```python
from build123d import *

# Parameters (mm, degrees)
SKETCH2_R                        = 3
BOSS_EXTRUDE1_DEPTH              = 25
SKETCH5_W                        = 200
SKETCH5_H                        = 44
CUT_EXTRUDE1_DEPTH               = 8
SENSORMODULE_BOTTOMMIDDLEE_DEPTH = 4.5
SKETCH12_W                       = 247.875067181
SKETCH12_H                       = 102.432022038
CUT_EXTRUDE2_DEPTH               = 14
SKETCH14_W                       = 9.40210165
SKETCH14_H                       = 8
SKETCH14_W_2                     = 8.199489831
BOSS_EXTRUDE2_DEPTH              = 48
FILLET1_R                        = 3
FILLET2_R                        = 3
SKETCH15_W                       = 3.793616894
SKETCH15_H                       = 8.666666667
SKETCH15_H_2                     = 8.666666666
BOSS_EXTRUDE3_DEPTH              = 8
SKETCH16_W                       = 3.793616895
SKETCH16_H                       = 8.666666667
SKETCH16_H_2                     = 8.666666666
BOSS_EXTRUDE4_DEPTH              = 10


with BuildPart() as part:
    # Sketch2 → Boss-Extrude1 (new body)
    with BuildSketch(Plane(origin=(0, 0, 0), x_dir=(1, 0, 0), z_dir=(0, 1, 0))):
        with BuildLine():
            Line((-33, -35), (33, -35))
            ThreePointArc((33, -35), (36.535533906, -33.535533906), (38, -30))
            Line((38, -30), (38, 30))
            ThreePointArc((38, 30), (36.535533906, 33.535533906), (33, 35))
            Line((33, 35), (-33, 35))
            ThreePointArc((-33, 35), (-36.535533906, 33.535533906), (-38, 30))
            Line((-38, 30), (-38, -30))
            ThreePointArc((-38, -30), (-36.535533906, -33.535533906), (-33, -35))
        make_face()
        with Locations((-33, 30)):
            Circle(SKETCH2_R, mode=Mode.SUBTRACT)
        with Locations((-33, -30)):
            Circle(SKETCH2_R, mode=Mode.SUBTRACT)
        with Locations((33, 30)):
            Circle(SKETCH2_R, mode=Mode.SUBTRACT)
        with Locations((33, -30)):
            Circle(SKETCH2_R, mode=Mode.SUBTRACT)
    extrude(amount=BOSS_EXTRUDE1_DEPTH)

    # Sketch5 → Cut-Extrude1 (cut)
    with BuildSketch(Plane(origin=(0, 25, 0), x_dir=(1, 0, 0), z_dir=(0, 1, 0))):
        Rectangle(SKETCH5_W, SKETCH5_H)
    extrude(amount=-CUT_EXTRUDE1_DEPTH, mode=Mode.SUBTRACT)

    # Sketch6 → SensorModule(bottomMiddlee) (add)
    with BuildSketch(Plane(origin=(87.622938947, 17, 0), x_dir=(1, 0, 0), z_dir=(0, 1, 0))):
        Polygon((-106.839454309, 15.5), (-75.839454309, 15.5), (-75.839454309, 7.8), (-68.839454309, 7.8), (-68.839454309, -7.4), (-75.839454309, -7.4), (-75.839454309, -15.5), (-106.839454309, -15.5), align=None)
    extrude(amount=SENSORMODULE_BOTTOMMIDDLEE_DEPTH)

    # Sketch12 → Cut-Extrude2 (cut)
    with BuildSketch(Plane.XZ):
        with Locations((-0.926975658, -6.36803857)):
            Rectangle(SKETCH12_W, SKETCH12_H)
    extrude(amount=-CUT_EXTRUDE2_DEPTH, mode=Mode.SUBTRACT)

    # Sketch14 → Boss-Extrude2 (add)
    with BuildSketch(Plane.XY.offset(-22)):
        with Locations((-33.298949175, 21)):
            Rectangle(SKETCH14_W, SKETCH14_H)
        with Locations((33.900255085, 21)):
            Rectangle(SKETCH14_W_2, SKETCH14_H)
    extrude(amount=BOSS_EXTRUDE2_DEPTH)

    # Fillet1
    fillet1_edges = [part.edges().sort_by_distance(p)[0] for p in [
        (0.601305909, 17, -22),
    ]]
    fillet(fillet1_edges, radius=FILLET1_R)

    # Fillet2
    fillet2_edges = [part.edges().sort_by_distance(p)[0] for p in [
        (0.601305909, 17, 22),
    ]]
    fillet(fillet2_edges, radius=FILLET2_R)

    # Sketch15 → Boss-Extrude3 (add)
    with BuildSketch(Plane(origin=(3.489394794, 17, 0), x_dir=(1, 0, 0), z_dir=(0, 1, 0))):
        with Locations((-27.729371665, 12.666666666)):
            Rectangle(SKETCH15_W, SKETCH15_H)
        with Locations((-27.729371665, 0)):
            Rectangle(SKETCH15_W, SKETCH15_H_2)
        with Locations((-27.729371665, -12.666666666)):
            Rectangle(SKETCH15_W, SKETCH15_H)
    extrude(amount=BOSS_EXTRUDE3_DEPTH)

    # Sketch16 → Boss-Extrude4 (add)
    with BuildSketch(Plane(origin=(51.94610351, 25, 9.710186869), x_dir=(1, 0, 0), z_dir=(0, 1, 0))):
        with Locations((-27.906397887, 22.722574296)):
            Rectangle(SKETCH16_W, SKETCH16_H)
        with Locations((-27.906397887, 10.055907629)):
            Rectangle(SKETCH16_W, SKETCH16_H_2)
        with Locations((-27.906397887, -2.610759038)):
            Rectangle(SKETCH16_W, SKETCH16_H)
    extrude(amount=-BOSS_EXTRUDE4_DEPTH)


solid = part.part
```
Model file for the job. Use its own axes, mm. A direction names the side the tool comes from. Give positions to 0.01 mm unless a question says otherwise; leave off trailing zeros. Write each loop counter-clockwise with the first axis right and the second up, starting at its lowest first coordinate (ties: lowest second). Pieces come first, ordered by that corner, then holes. Notation, with made-up numbers: M 36.5,78 L 83.5,78 A20 cw 83.5,101 Z; hole C -5,23 d11. An arc over 180 degrees is marked long. Use a Markdown table: item, result.
1) Cut at B-B (x = 9.5). List the corners of the cut face in (y, z).
Responses:
| item | result |
|---|---|
| outline | M 14,-35 L 25,-35 L 25,-22 L 20,-22 A3 cw 17,-19 L 17,-15.5 L 21.5,-15.5 L 21.5,15.5 L 17,15.5 L 17,19 A3 cw 20,22 L 25,22 L 25,35 L 14,35 Z |
2) Pin check, flat tip, straight feed: pin 1 (7 mm diameter, centred on x = -33, z = -30, fed in from +Y). Stop position of the tip, or through.
Responses:
| item | result |
|---|---|
| pin 1 | stops at y = 25 |
3) Drill centre lines: line 1 (Z direction, x = -33, y = 16.5); line 2 (X direction, y = 21.25, z = 15); line 3 (X direction, y = 22.75, z = 30). Where is each one in solid material? Low to high. Write a range as from..to.
Responses:
| item | result |
|---|---|
| line 1 | z = -35..-33, -27..27, 33..35 |
| line 2 | x = -38..-28.6, -26.14..-22.34, -19.22..11.78, 22.14..25.94, 29.8..38 |
| line 3 | x = -38..-36, -30..30, 36..38 |
4) Pull direction X, two halves, no side cores. Call faces 1 (the cylindrical face through (-36, 19, -34)), 2 (the flat face through (24, 25, 12)), 3 (the flat face through (22.143, 21, -13)): +X half, -X half, draft (parallel to the pull), parting line (faces both ways), or undercut.
Responses:
| item | result |
|---|---|
| face 1 | -X half |
| face 2 | draft |
| face 3 | undercut |
5) Cut at D-D (x = 27). List the corners of the cut face in (y, z).
Responses:
| item | result |
|---|---|
| outline | M 14,-35 L 25,-35 L 25,-22 L 20,-22 A3 cw 17,-19 L 17,19 A3 cw 20,22 L 25,22 L 25,35 L 14,35 Z |
6) Cut at C-C (x = -23.5). List the corners of the cut face in (y, z), and give its area (3 significant figures).
Responses:
| item | result |
|---|---|
| outline | M 14,-35 L 25,-35 L 25,-22 L 20,-22 A3 cw 17,-19 L 17,-17 L 25,-17 L 25,-8.33 L 17,-8.33 L 17,-4.33 L 25,-4.33 L 25,4.33 L 17,4.33 L 17,8.33 L 25,8.33 L 25,17 L 17,17 L 17,19 A3 cw 20,22 L 25,22 L 25,35 L 14,35 Z |
| area | 630 mm2 |
7) Cut at A-A (y = 15.5). List the corners of the cut face in (x, z), and give its area (3 significant figures).
Responses:
| item | result |
|---|---|
| outline | M -38,-30 A5 ccw -33,-35 L 33,-35 A5 ccw 38,-30 L 38,30 A5 ccw 33,35 L -33,35 A5 ccw -38,30 Z; hole C -33,-30 d6; hole C -33,30 d6; hole C 33,-30 d6; hole C 33,30 d6 |
| area | 5,190 mm2 |
8) Tool access for faces 4 (the flat face through (-24, 21, -4.333)), 5 (the flat face through (-1, 14, 0)): list every direction of +Z, -Z, +X, -X, +Y, -Y with a clear straight run to the whole face (end or side of a thin tool).
Responses:
| item | result |
|---|---|
| face 4 | +Y |
| face 5 | +Z, -Z, +X, -X, -Y |
